Geometry: final body of the model. Coordinates: model frame, mm. A direction names the side the tool comes from. Round coordinates to 2 decimals unless told otherwise and drop trailing zeros. Loops run counter-clockwise (first coordinate to the right, second up) from the corner with the lowest first, then second, coordinate; pieces in that order, holes last. Notation, with made-up numbers: (-25, 1.25) - (1, 1.25) arc R14 ccw to (1, 13.25) - close; hole circle Ø2 at (32, 12.25). An arc over 180 degrees is marked (long way). Answer in a Markdown table with one row per item. Add a question column.
from build123d import *

# Parameters (mm, degrees)
SKETCH1_R                      = 79.375
BOSS_EXTRUDE1_DEPTH            = 3.175
SKETCH5_R                      = 11
CUT_EXTRUDE1_DEPTH             = 2.5
SKETCH6_R                      = 5
CUT_EXTRUDE2_DEPTH             = 113.432663181
CBORE_FOR_M2_SHCS1_D           = 2.2
CBORE_FOR_M2_SHCS1_DEPTH       = 6
CBORE_FOR_M2_SHCS1_CBORE_D     = 4.4
CBORE_FOR_M2_SHCS1_CBORE_DEPTH = 2
CBORE_FOR_M2_SHCS1_TIP         = 0.660946681
M4_CLEARANCE_HOLE1_D           = 4.5
M5_CLEARANCE_HOLE1_D           = 5.5
CHAMFER1_SIZE                  = 2.5


with BuildPart() as part:
    # Sketch1 → Boss-Extrude1 (new, symmetric)
    with BuildSketch(Plane(origin=(0, 0, 0), x_dir=(1, 0, 0), z_dir=(0, 1, 0))):
        with Locations(Location((0, 0, 0), (0, 0, 270))):
            Circle(SKETCH1_R)
    extrude(amount=BOSS_EXTRUDE1_DEPTH, both=True)

    # Sketch5 → Cut-Extrude1 (cut)
    with BuildSketch(Plane(origin=(0, 3.175, 0), x_dir=(1, 0, 0), z_dir=(0, 1, 0))):
        with Locations(Location((0, 0, 0), (0, 0, 270))):
            Circle(SKETCH5_R)
    extrude(amount=-CUT_EXTRUDE1_DEPTH, mode=Mode.SUBTRACT)

    # Sketch6 → Cut-Extrude2 (cut, through all)
    with BuildSketch(Plane(origin=(0, 3.175, 0), x_dir=(1, 0, 0), z_dir=(0, 1, 0))):
        with Locations(Location((0, 0, 0), (0, 0, 270))):
            Circle(SKETCH6_R)
    extrude(amount=-CUT_EXTRUDE2_DEPTH, mode=Mode.SUBTRACT)

    # CBORE for M2 SHCS1
    with Locations(Plane(origin=(0, 0.675, 0), x_dir=(1, 0, 0), z_dir=(0, 1, 0))):
        with Locations((-5.65685425, 5.65685425), (0, 8), (5.65685425, 5.65685425), (8, 0), (5.65685425, -5.65685425), (0, -8), (-5.65685425, -5.65685425), (-8, 0)):
            CounterBoreHole(CBORE_FOR_M2_SHCS1_D / 2, CBORE_FOR_M2_SHCS1_CBORE_D / 2, CBORE_FOR_M2_SHCS1_CBORE_DEPTH, depth=CBORE_FOR_M2_SHCS1_DEPTH)
            with Locations((0, 0, -(CBORE_FOR_M2_SHCS1_DEPTH + CBORE_FOR_M2_SHCS1_TIP / 2))):  # 118° drill point
                Cone(0, CBORE_FOR_M2_SHCS1_D / 2, CBORE_FOR_M2_SHCS1_TIP, mode=Mode.SUBTRACT)

    # M4 Clearance Hole1 (through all)
    with Locations(Plane(origin=(0, 3.175, 0), x_dir=(1, 0, 0), z_dir=(0, 1, 0))):
        with Locations((19.05, -44.388212048), (-19.05, -44.388212048)):
            Hole(M4_CLEARANCE_HOLE1_D / 2)

    # M5 Clearance Hole1 (through all)
    with Locations(Plane(origin=(0, 3.175, 0), x_dir=(1, 0, 0), z_dir=(0, 1, 0))):
        with Locations((-33.6688086, 31.567387952), (-14.6188086, 31.567387952), (4.4311914, 31.567387952), (-15.875, -19.249706448), (15.875, -19.249706448)):
            Hole(M5_CLEARANCE_HOLE1_D / 2)

    # Chamfer1
    chamfer1_edges = [part.edges().sort_by_distance(p)[0] for p in [
        (0, 3.175, -11),
    ]]
    chamfer(chamfer1_edges, length=CHAMFER1_SIZE - 0.0001)  # a hair under: the kernel refuses the full size


solid = part.part
1) Section B-B, the plane z = 28.5. Return the cut outline in (x, y) (3 decimals).
2) Pull-direction query (X, two-part tool) for faces 3 (the flat face through (1, 3.175, 17)), 4 (the flat face through (-7, -1.325, -5)); classes: pulls with the +X half, pulls with the -X half, needs draft (parallel to the pull), parting line crosses it, or undercut.
3) Section A-A, the plane x = -55.5. Return the cut outline in (y, z) (3 decimals).
4) Reachability of faces 1 (the flat face through (1, -3.175, 17)), 2 (the flat face through (-1, -1.325, -9)) from +Z, -Z, +X, -X, +Y, -Y: full face, straight path, thin tool, end or side. Return the list, or none.
5) Contact query for flat-ended pins moving along their axis: pin 1 Ø6.5 at (x, z) = (-14.62, -31.57) entering from +Y (3 decimals); pin 2 Ø2 at (x, y) = (-8, 0) entering from -Z; pin 3 Ø4.5 at (x, z) = (-15.88, 19.25) entering from -Y; pin 4 Ø1.5 at (y, z) = (-1, 29.5) entering from -X. Output: stop coordinate, or through.
6) Material intervals for line 1 along X through (y, z) = (-0.75, -5.5); line 2 along X through (y, z) = (-1.25, 44.5); line 3 along Z through (x, y) = (-15.5, -3), sorted ascending. Write a range as from..to.
Evaluation:
| question | item | result |
|---|---|---|
| 1 | outline | (-74.082, -3.175) - (74.082, -3.175) - (74.082, 3.175) - (-74.082, 3.175) - close |
| 2 | face 3 | needs draft |
| 2 | face 4 | undercut |
| 3 | outline | (-3.175, -56.746) - (3.175, -56.746) - (3.175, 56.746) - (-3.175, 56.746) - close |
| 4 | face 1 | +Z, -Z, +X, -X, -Y |
| 4 | face 2 | +Y |
| 5 | pin 1 | stops at y = 3.175 |
| 5 | pin 2 | stops at z = -79.07 |
| 5 | pin 3 | passes through |
| 5 | pin 4 | stops at x = -73.99 |
| 6 | line 1 | x = -79.18..-7.85, -3.46..3.46, 7.85..79.18 |
| 6 | line 2 | x = -65.73..-21.3, -16.8..16.8, 21.3..65.73 |
| 6 | line 3 | z = -77.85..-34.17, -28.96..16.53, 21.97..77.85 |
